Check sheet for the modelled part. Datum: model origin and axes. Units: mm. A direction names the side the tool comes from. Give positions to 0.01 mm unless a question says otherwise; leave off trailing zeros. Order: outer loops, then holes, each group sorted by start corner. A loop starts at its lowest first (then second) coordinate and runs counter-clockwise, first axis right, second up. Notation, with made-up numbers: M 0.5,1.25 L 41.5,1.25 A27 ccw 41.5,18.25 Z; hole C 68,5.5 d7. An arc over 180 degrees is marked long. Return JSON: item names as keys, results as strings. Group by question number.
Autodesk Inventor part; units mm, degrees
ref_plane "YZ Plane" through (0, 0, 0) normal (1, 0, 0) x (0, 1, 0)
ref_plane "XZ Plane" through (0, 0, 0) normal (0, 1, 0) x (-1, 0, 0)
ref_plane "XY Plane" through (0, 0, 0) normal (0, 0, 1) x (1, 0, 0)
ref_plane "Work Plane1" through (88.0411, 0, -4.3553) normal (0, 1, 0) x (-1, 0, 0)
sketch "Sketch1" plane through (88.0411, 0, -4.3553) normal (0, 1, 0) x (-1, 0, 0)
  line L0 (58.171, -0.729) -> (56.0977, -0.729)
  line L1 (56.0977, -0.729) -> (54.0127, -0.3924)
  line L2 (54.0127, -0.3924) -> (50.0902, -0.0001)
  line L3 (50.0902, -0.0001) -> (48.159, -0.0001)
  line L4 (48.159, -0.0001) -> (48.159, -0.9194)
  line L5 (48.159, -0.9194) -> (46.281, -0.9194)
  line L6 (46.281, -0.9194) -> (44.3734, -0.6114)
  line L7 (44.3734, -0.6114) -> (42.5702, -0.4904)
  line L8 (42.5702, -0.4904) -> (38.7992, -0.4904)
  line L9 (38.7992, -0.4904) -> (36.9307, -0.729)
  line L10 (36.9307, -0.729) -> (35.0405, -1.2743)
  line L11 (35.0405, -1.2743) -> (32.7869, -1.7551)
  line L12 (32.7869, -1.7551) -> (31.1597, -2.2246)
  line L13 (31.1597, -2.2246) -> (29.2392, -2.5119)
  line L14 (29.2392, -2.5119) -> (25.7568, -2.5119)
  line L15 (25.7568, -2.5119) -> (22.1476, -1.9292)
  line L16 (22.1476, -1.9292) -> (20.1771, -1.9292)
  line L17 (20.1771, -1.9292) -> (20.1771, -3.0939)
  line L18 (20.1771, -3.0939) -> (15.2755, -3.0939)
  line L19 (15.2755, -3.0939) -> (12.2384, -2.6036)
  line L20 (12.2384, -2.6036) -> (10.4528, -2.6036)
  line L21 (10.4528, -2.6036) -> (8.2143, -2.8887)
  line L22 (8.2143, -2.8887) -> (6.4213, -2.7683)
  line L23 (6.4213, -2.7683) -> (6.4213, -2.4041)
  line L24 (6.4213, -2.4041) -> (3.9663, -2.6036)
  line L25 (3.9663, -2.6036) -> (1.931, -2.8628)
  line L26 (1.931, -2.8628) -> (-0.0002, -2.7332)
  line L27 (-0.0002, -2.7332) -> (-0.0002, -9.8132)
  line L28 (-0.0002, -9.8132) -> (-6.1102, -9.8132)
  line L29 (-6.1102, -9.8132) -> (-6.1102, -18.749)
  line L30 (-6.1102, -18.749) -> (58.171, -18.749)
  line L31 (58.171, -18.749) -> (58.171, -0.729)
  line L32 (58.171, -0.0001) -> (-0.0002, -0.0001)
  line L33 (-0.0002, -0.0001) -> (-0.0002, -2.7332)
  line L34 (-0.0002, -2.7332) -> (58.171, -2.7332)
  line L35 (58.171, -2.7332) -> (58.171, -0.0001)
  line L36 (-0.0002, -0.0001) -> (81.9998, -0.0001)
  line L37 (81.9998, -0.0001) -> (81.9998, 1.9999)
  line L38 (81.9998, 1.9999) -> (-0.0002, 1.9999)
  line L39 (-0.0002, 1.9999) -> (-0.0002, -0.0001)
  point P0 (88.0411, 4.3553)
  point P1 (2.9486, -2.7332)
  point P2 (6.4213, -2.7332)
  point P3 (9.4352, -2.7332)
  point P4 (31.9998, 9.1499)
  point P5 (20.1771, -2.7332)
  point P6 (13.0411, -2.7332)
  point P7 (48.159, -0.0001)
  point P8 (58.171, -2.7332)
  point P9 (50.0902, -0.0001)
  dimension "d0" = 2
  dimension "d13" = 50
extrude "Extrusion1" add sketch "Sketch1" along normal blind 50 contours L31 L34 L17 L16 L15 L14 L13 L12 L11 L10 L9 L8 L7 L6 L5 L4 L3 L2 L1 L0 | L0 L1 L2 L32 L35 | L32 L3 L39 L38 L37 L36 | L34 L19 L20 L21 L23 L24 L25 L33 L32 L4 L5 L6 L7 L8 L9 L10 L11 L12 L13 L14 L15 L16 L17 | L34 L21 L20 L19 | L21 L22 L23 L34 | L34 L25 L24 L23 | L34 L25 L26
sketch "Sketch2" plane through (6.0413, 0, -2.3554) normal (0, 0, 1) x (1, 0, 0)
  line L0 (2.0733, 0) -> (0, 0)
  line L1 (82, 0) -> (82, 50)
  line L2 (0, 0) -> (82, 0)
  line L3 (82, 0) -> (82, 3)
  line L4 (82, 3) -> (0, 3)
  line L5 (0, 3) -> (0, 0)
  circle A0 centre (50, 40.5) radius 32 construction
  line L6 (58.1712, -304.8) -> (58.1712, 304.8) construction
  circle A1 centre (50, 40.5) radius 3.925
  circle A2 centre (50, 40.5) radius 1.925
  point P0 (-6.0413, 0)
  point P1 (10, 40.5)
  dimension "d3" = 3
  dimension "d6" = 64
  dimension "d7" = 37.5
  dimension "d8" = 32
  dimension "d9" = 7.85
  dimension "d10" = 2
  dimension "d14" = 40
extrude "Extrusion2" add sketch "Sketch2" along normal blind 7 contours L0 L5 L4 L1 L2
extrude "Extrusion3" add sketch "Sketch2" along normal blind 7.15 contours A1
equation "\"t\" = 0.15"
properties part number "backCase"
1) Depth check by flat-ended pin: P1, Ø2, axis at y = 21.5, z = -6, coming from the -X side; P2, Ø10, axis at x = 24.5, y = 44.5, coming from the +Z side; P3, Ø3.5, axis at x = 61.5, y = 1.5, coming from the +Z side; P4, Ø6, axis at x = 56.04, y = 40.5, coming from the +Z side. Enter the tip coordinate at first touch or a pass-through.
2) Sectioned sample at A-A on z = 2.75. Record the boundary of the cut face in (x, y) (3 decimals).
3) Release check for a two-part mould opening along Y. For faces 1 (the face through (55, 25, -7.088)), 2 (the face through (57, 50, -5)), 3 (the face through (56, 40, -2.355)), 4 (the face through (52.12, 40.33, 1.17)) record: released by +Y, released by -Y, zero draft, split by the parting line, or undercut.
4) Material ranges on line 1 along X through (y, z) = (44, -6.5); line 2 along Z through (x, y) = (69.5, 30); line 3 along Y through (x, z) = (58, 2), recorded low to high.
5) Sectioned sample at D-D on x = 33.5. Record the boundary of the cut face in (y, z), then the cut area to 3 significant figures.
6) Tool access check on faces 5 (the face through (88.041, 25, -4)), 6 (the face through (18, 25, -4.355)), 7 (the face through (80.711, 24.65, -7.185)), 8 (the face through (57.82, 41.24, 1.17)). Record the directions out of +Z, -Z, +X, -X, +Y, -Y that give a thin tool (end or side, any length) a straight path to the whole face; none if there is none.
7) Sectioned sample at C-C on z = -5.5. Record the boundary of the cut face in (x, y).
Reply:
{
 "1": {"P1": "x = 29.87", "P2": "z = -2.36", "P3": "z = 4.64", "P4": "z = 4.79"},
 "2": {"outline": "M 6.041,0 L 88.041,0 L 88.041,3 L 6.041,3 Z; C 56.041,40.5 d7.85; hole C 56.041,40.5 d3.85"},
 "3": {"face 1": "zero draft", "face 2": "released by +Y", "face 3": "undercut", "face 4": "undercut"},
 "4": {"line 1": "29.87 to 88.04", "line 2": "-7.09 to -2.36", "line 3": "0 to 3, 37.1 to 43.9"},
 "5": {"outline": "M 0,-7.09 L 50,-7.09 L 50,-2.36 L 3,-2.36 L 3,4.64 L 0,4.64 Z", "area": "258 mm^2"},
 "6": {"face 5": "+Z, -Z, +X, +Y, -Y", "face 6": "-Z, -X, +Y, -Y", "face 7": "-Z, +Y, -Y", "face 8": "+Z"},
 "7": {"outline": "M 29.87,0 L 88.04,0 L 88.04,50 L 29.87,50 Z"}
}
